Can you work these out from the drawing? Everything is in mm from the part's minimum corner. Give positions to 0.01 mm unless a question says otherwise; leave off trailing zeros. Loops run counter-clockwise (first coordinate to the right, second up) from the corner with the lowest first, then second, coordinate; pieces in that order, holes last. Notation, with made-up numbers: M -35.75,17 L 12.25,17 A32 ccw 12.25,56 Z; hole C 83,-14.75 d3. An arc over 180 degrees is marked long. Use CSV: the item, a comma, the result in double quotes.
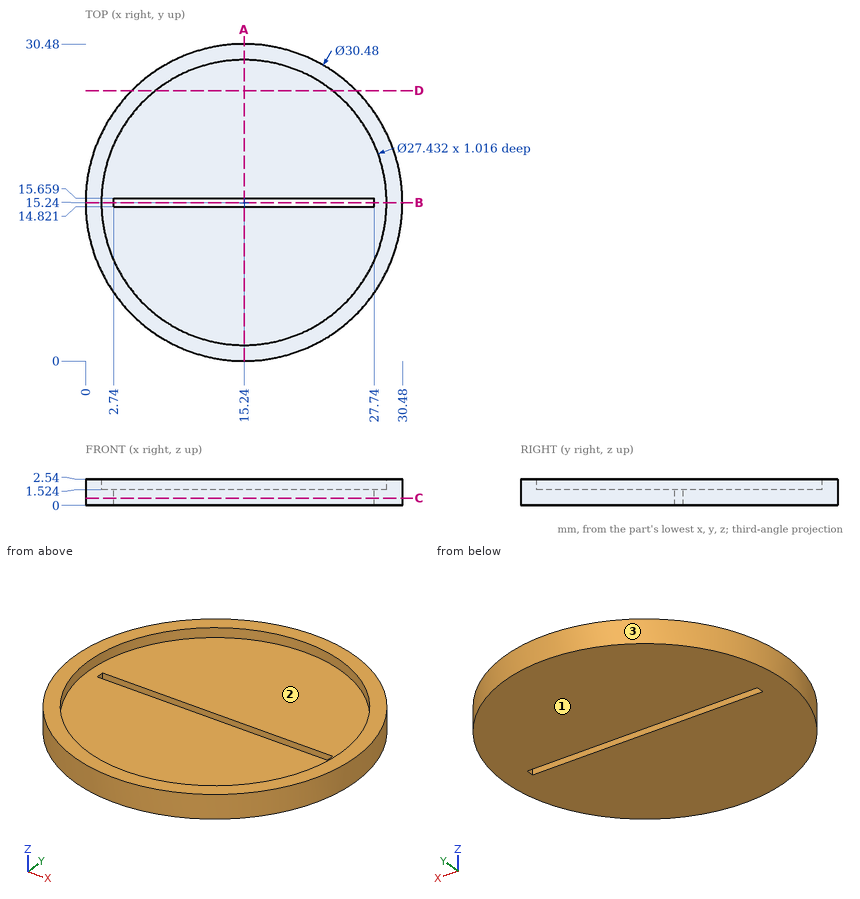
Q1. I want a section at C-C, the plane z = 0.7. Please give me the cut outline in (x, y).
Model answer:
outline,"C 15.24,15.24 d30.48; hole M 2.74,14.82 L 27.74,14.82 L 27.74,15.66 L 2.74,15.66 Z"
Q2. I want a section at D-D, the plane y = 26. Please give me the cut outline in (x, z).
Model answer:
outline,"M 4.45,0 L 26.03,0 L 26.03,2.54 L 23.75,2.54 L 23.75,1.52 L 6.73,1.52 L 6.73,2.54 L 4.45,2.54 Z"
Q3. I want a section at A-A, the plane x = 15.24. Please give me the cut outline in (y, z), then the cut area to 3 significant figures.
Model answer:
outline,"M 0,0 L 14.82,0 L 14.82,1.52 L 1.52,1.52 L 1.52,2.54 L 0,2.54 Z; M 15.66,0 L 30.48,0 L 30.48,2.54 L 28.96,2.54 L 28.96,1.52 L 15.66,1.52 Z"
area,"48.3 mm2"
Q4. Please list where these lines run through material, in increasing order: L1, parallel to X at y = 15, z = 1.05; L2, parallel to Y at x = 15.24, z = 2.15; L3, parallel to Z at x = 19.5, y = 11. Write a range as from..to.
Model answer:
L1,"0..2.74, 27.74..30.48"
L2,"0..1.52, 28.96..30.48"
L3,"0..1.52"
Q5. I want a section at B-B, the plane y = 15.24. Please give me the cut outline in (x, z).
Model answer:
outline,"M 0,0 L 2.74,0 L 2.74,1.52 L 1.52,1.52 L 1.52,2.54 L 0,2.54 Z; M 27.74,0 L 30.48,0 L 30.48,2.54 L 28.96,2.54 L 28.96,1.52 L 27.74,1.52 Z"
Q6. I'm going to push flat-ended pins straight in: P1, Ø6, axis at x = 13.5, y = 9, coming from the +Z side; P2, Ø1.2, axis at x = 18.5, z = 0.5, coming from the +Y side. Where does each tip first touch, or does it pass through?
Model answer:
P1,"z = 1.52"
P2,"y = 30.25"
Q7. If we mould it in two halves opening along X, with no side actions, what happens to the marked faces 1, 2 and 3? For each: released by +X, released by -X, zero draft, split by the parting line, or undercut.
Model answer:
face 1,"zero draft"
face 2,"undercut"
face 3,"split by the parting line"
